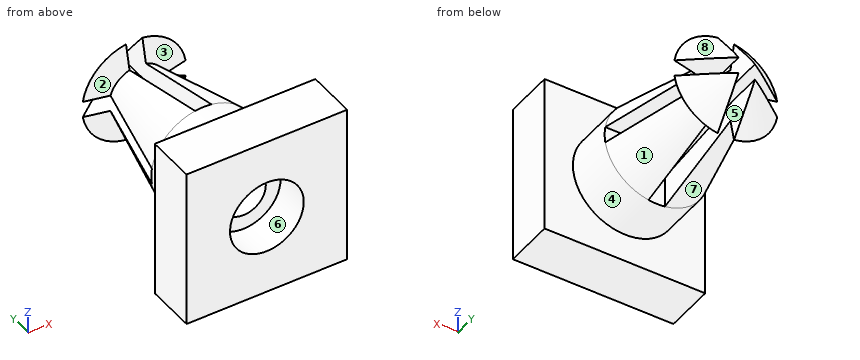
```python
from build123d import *

# Parameters (mm, degrees)
F0_W     = 9.8
F0_H     = 9.8
F0_R     = 2.75
F3_DEPTH = 1.5
F5_START = -4.5
F4_W     = 1
F4_H     = 4.5
F4_H_2   = 1
F4_W_2   = 4.5
F5_DEPTH = 20.5


# Not quite as in the source:
# - a feature names something its author has since deleted; it is built from what else it names


with BuildPart() as f2:
    # F1 (on Right) → F2 (revolve)
    with BuildSketch(Plane.YZ):
        Polygon((4.5, 3.175), (-1.5, 3.175), (-1.5, 2.25), (0.6892941068, 2.25), (0.6892941068, 1.35), (4.0952532458, 1.35), (13.1507472004, 0.5), (11.0196430301, 3.175), (10.6847711314, 1.7358662147), align=None)
    revolve(axis=Axis((0, 11.4737532458, 0), (0, 1, 0)))

    # F0 (on Front) → F3 (join, symmetric)
    with BuildSketch(Plane.XZ):
        Rectangle(F0_W, F0_H)
        Circle(F0_R, mode=Mode.SUBTRACT)
    extrude(amount=F3_DEPTH, both=True)

    # F4 (on Front) → F5 (cut)
    with BuildSketch(Plane.XZ.offset(F5_START)):
        with Locations((0, 2.75)):
            Rectangle(F4_W, F4_H)
        Rectangle(F4_W, F4_H_2)
        with Locations((-2.75, 0)):
            Rectangle(F4_W_2, F4_H_2)
        with Locations((2.75, 0)):
            Rectangle(F4_W_2, F4_H_2)
        with Locations((0, -2.75)):
            Rectangle(F4_W, F4_H)
    extrude(amount=-F5_DEPTH, mode=Mode.SUBTRACT)


solid = f2.part
```
Model file for the job. Use its own axes, mm. Face numbers are marked on the shaded views. A direction names the side the tool comes from. Coordinates: 2 decimals unless noted, no trailing zeros. Order: outer loops, then holes, each group sorted by start corner. A loop starts at its lowest first (then second) coordinate and runs counter-clockwise, first axis right, second up. Notation, with made-up numbers: (63.5, 43) - (105.5, 43) arc R29 cw to (105.5, 69) - close; hole circle Ø1 at (-37.5, 4). An arc over 180 degrees is marked (long way). Return JSON: item names as keys, results as strings. Group by question number.
1) Saw through at D-D, the plane y = 0. Write the cut outline in (x, z).
2) Saw through at C-C, the plane z = 0. Write the cut outline in (x, y) (3 decimals), plus the area to 3 significant figures.
3) Saw through at A-A, the plane y = 6.25. Write the cut outline in (x, z).
4) Mould opens along Z. For the marked faces 6, 7 and 8 say: released by +Z, released by -Z, zero draft, split by the parting line, or undercut.
5) Probe line 1 (X direction, y = 1.4, z = 0); line 2 (X direction, y = -0.95, z = 0); line 3 (Y direction, x = 4, z = 0.5). List the from-to ranges inside material, lowest first. Write a range as from..to.
6) Tool access for the marked faces 1, 2, 3, 4 and 5: list every direction of +Z, -Z, +X, -X, +Y, -Y with a clear straight run to the whole face (end or side of a thin tool).
7) Saw through at B-B, the plane x = 0. Write the cut outline in (y, z) (3 decimals), plus the area to 3 significant figures.
8) Flat gauge pins, fed straight in: P1, Ø0.8, axis at x = -2, z = 0, coming from the +Y side; P2, Ø2, axis at x = -1, z = 0.5, coming from the -Y side; P3, Ø4, axis at x = -1.5, z = 4, coming from the +Y side. Where does each tip first touch, or does it go through?
Values found:
{
 "1": {"outline": "(-4.9, -4.9) - (4.9, -4.9) - (4.9, 4.9) - (-4.9, 4.9) - close; hole circle Ø4.5 at (0, 0)"},
 "2": {"outline": "(-4.9, -1.5) - (-2.25, -1.5) - (-2.25, 0.689) - (-1.35, 0.689) - (-1.35, 4.095) - (-1.312, 4.5) - (-3.175, 4.5) - (-3.175, 1.5) - (-4.9, 1.5) - close; (1.312, 4.5) - (1.35, 4.095) - (1.35, 0.689) - (2.25, 0.689) - (2.25, -1.5) - (4.9, -1.5) - (4.9, 1.5) - (3.175, 1.5) - (3.175, 4.5) - close", "area": "28.3 mm²"},
 "3": {"outline": "(-2.72, -0.5) arc R2.77 ccw to (-0.5, -2.72) - (-0.5, -1.03) arc R1.15 cw to (-1.03, -0.5) - close; (-2.72, 0.5) - (-1.03, 0.5) arc R1.15 cw to (-0.5, 1.03) - (-0.5, 2.72) arc R2.77 ccw to start; (0.5, -2.72) arc R2.77 ccw to (2.72, -0.5) - (1.03, -0.5) arc R1.15 cw to (0.5, -1.03) - close; (0.5, 1.03) arc R1.15 cw to (1.03, 0.5) - (2.72, 0.5) arc R2.77 ccw to (0.5, 2.72) - close"},
 "4": {"face 6": "undercut", "face 7": "released by -Z", "face 8": "released by +Z"},
 "5": {"line 1": "x = -4.9..-1.35, 1.35..4.9", "line 2": "x = -4.9..-2.25, 2.25..4.9", "line 3": "y = -1.5..1.5"},
 "6": {"face 1": "-Z, +X", "face 2": "+Z, -X", "face 3": "+Z, +X", "face 4": "+Y", "face 5": "+Z, -Z, +Y"},
 "7": {"outline": "(-1.5, -4.9) - (1.5, -4.9) - (1.5, -3.175) - (4.5, -3.175) - (4.5, -1.312) - (4.095, -1.35) - (0.689, -1.35) - (0.689, -2.25) - (-1.5, -2.25) - close; (-1.5, 2.25) - (0.689, 2.25) - (0.689, 1.35) - (4.095, 1.35) - (4.5, 1.312) - (4.5, 3.175) - (1.5, 3.175) - (1.5, 4.9) - (-1.5, 4.9) - close", "area": "28.3 mm²"},
 "8": {"P1": "stops at y = 4.5", "P2": "stops at y = 0.69", "P3": "stops at y = 11.74"}
}
